from build123d import *

# Parameters (mm, degrees)
SKETCH_1_R      = 1.5
SKETCH_1_R_2    = 3.85
EXTRUDE_1_DEPTH = 3


with BuildPart() as part:
    # 草圖1 → 填料-伸長1 (new body)
    with BuildSketch(Plane.XY):
        with BuildLine():
            Line((-1.088072116, -16.755807147), (45.162709199, -16.755807147))
            ThreePointArc((45.162709199, -16.755807147), (56.790010388, -3.27850574), (41.753879517, 6.247592861))
            ThreePointArc((41.753879517, 6.247592861), (39.868271169, 5.774911831), (37.945680681, 5.487523562))
            ThreePointArc((37.945680681, 5.487523562), (31.659768337, 5.100288193), (25.363940234, 5.25901355))
            ThreePointArc((25.363940234, 5.25901355), (12.306009375, 11.647221283), (7.023040081, 25.190078877))
            Line((7.023040081, 25.190078877), (7.023039951, 29.795438865))
            ThreePointArc((7.023039951, 29.795438865), (-4.532515913, 41.350994164), (-16.088071721, 29.795438809))
            Line((-16.088071721, 29.795438809), (-16.088072116, 20.328730687))
            Line((-16.088072116, 20.328730687), (-16.088072116, -1.755807147))
            ThreePointArc((-16.088072116, -1.755807147), (-11.694673834, -12.362408864), (-1.088072116, -16.755807147))
        make_face()
        with Locations((-4.532515885, 29.795438328)):
            Circle(SKETCH_1_R, mode=Mode.SUBTRACT)
        with Locations((45.162709199, -5.00153318)):
            Circle(SKETCH_1_R_2, mode=Mode.SUBTRACT)
        with Locations((-4.532515885, -5.00153318)):
            Circle(SKETCH_1_R, mode=Mode.SUBTRACT)
    extrude(amount=EXTRUDE_1_DEPTH)


solid = part.part
The model under review builds one solid part; all positions refer to its coordinate system, in mm. A direction names the side the tool comes from. Give positions to 0.01 mm unless a question says otherwise; leave off trailing zeros. Write each loop counter-clockwise with the first axis right and the second up, starting at its lowest first coordinate (ties: lowest second). Pieces come first, ordered by that corner, then holes. Notation, with made-up numbers: M -15,-14 L 6,-14 A21 ccw 6,-2 Z; hole C 35,1 d6. An arc over 180 degrees is marked long. One line per question, with ' | ' between items. Start each with the question number.
Item 1: For faces 5 (the flat face through (7.023, 27, 1)), 6 (the cylindrical face through (39.89, 5.78, 1.48)), 7 (the cylindrical face through (-11.811, -12.245, 1.479)), list the 3-axis set-ups (+Z, -Z, +X, -X, +Y, -Y) from which the entire face can be reached by the end or side of a thin tool; tool diameter is ignored.
Item 2: We need section B-B on z = 2.5. Write out the cut boundary in (x, y), plus the area to 3 significant figures.
Item 3: We need section D-D on x = 5. Write out the cut boundary in (y, z), plus the area to 3 significant figures.
Item 4: We need section C-C on y = 26. Write out the cut boundary in (x, z), plus the area to 3 significant figures.
Item 5: For pin 1 (1 mm diameter, centred on x = -6.5, z = 1, fed in from +Y); pin 2 (5 mm diameter, centred on x = -4.53, y = 29.8, fed in from +Z); pin 3 (1.5 mm diameter, centred on y = -11, z = 2.5, fed in from -X); pin 4 (1.5 mm diameter, centred on y = 28.5, z = 2, fed in from +X), all flat-tipped, find the tip position at first contact; note any pin that passes through.
Item 6: Draft analysis for pull direction Y (two halves, no side actions). For faces 1 (the cylindrical face through (48.719, -6.476, 1.479)), 2 (the flat face through (12, 6, 3)), 3 (the cylindrical face through (-4.86, 28.33, 1.48)), 4 (the cylindrical face through (12.45, 11.49, 1.48)), state which applies: released by +Y, released by -Y, zero draft, split by the parting line, or undercut.
Item 7: Wall thickness on line 1 (X direction, y = 30, z = 1.5); line 2 (X direction, y = -5.5, z = 2.15); line 3 (Y direction, x = -5, z = 1.6): over which ranges is each line inside the solid? List them lowest first. Write a range as from..to.
Item 8: We need section A-A on x = 46.5. Write out the cut boundary in (y, z), plus the area to 3 significant figures.
Results found:
1) face 5: +Z, -Z, +X, +Y | face 6: +Z, -Z, +Y | face 7: +Z, -Z, -X, -Y
2) outline: M -16.09,-1.76 A15 ccw -1.09,-16.76 L 45.16,-16.76 A11.75 ccw long 41.75,6.25 A20 cw 37.95,5.49 A72.64 cw 25.36,5.26 A20 cw 7.02,25.19 L 7.02,29.8 A11.56 ccw -16.09,29.8 Z; hole C -4.53,-5 d3; hole C -4.53,29.8 d3; hole C 45.16,-5 d7.7 | area: 2,320 mm2
3) outline: M -16.76,0 L 36.33,0 L 36.33,3 L -16.76,3 Z | area: 159 mm2
4) outline: M -16.09,0 L 7.02,0 L 7.02,3 L -16.09,3 Z | area: 69.3 mm2
5) pin 1: stops at y = 41.26 | pin 2: stops at z = 3 | pin 3: stops at x = -13.45 | pin 4: stops at x = 7.02
6) face 1: undercut | face 2: zero draft | face 3: undercut | face 4: released by +Y
7) line 1: x = -16.09..-6.02, -3.05..7.02 | line 2: x = -15.61..-5.95, -3.12..41.35, 48.98..56.91 | line 3: y = -16.24..-6.43, -3.58..28.37, 31.22..41.34
8) outline: M -16.68,0 L -8.61,0 L -8.61,3 L -16.68,3 Z; M -1.39,0 L 6.68,0 L 6.68,3 L -1.39,3 Z | area: 48.4 mm2
